```python
from build123d import *

# Parameters (mm, degrees)
BOSS_EXTRUDE1_DEPTH     = 25.4
CUT_EXTRUDE1_DEPTH      = 0.25399999999999945
CUT_EXTRUDE1_DEPTH_BACK = 3.8099999999999814
BOSS_EXTRUDE3_DEPTH     = 50.8
CUT_EXTRUDE3_DEPTH      = 38.1
SKETCH9_R               = 7.958201772862371
BOSS_EXTRUDE4_DEPTH     = 95.75799999999995
SKETCH11_W              = 88.91089611657237
SKETCH11_H              = 39.241441418777725
BOSS_EXTRUDE5_DEPTH     = 16.509999999999938
FILLET2_R               = 10
FILLET3_R               = 4.919999999999999


# Read off the part's stored shape, not the designer's step: Sweep1
with BuildPart() as part:
    # Sketch1 → Boss-Extrude1 (new body)
    with BuildSketch(Plane.XY):
        with BuildLine():
            Line((63.5, 77.01063829787236), (-63.5, 77.01063829787236))
            ThreePointArc((-63.5, 77.01063829787236), (-73.05346395858422, 73.05346395858422), (-77.01063829787236, 63.5))
            Line((-77.01063829787236, 63.5), (-77.01063829787236, -63.5))
            ThreePointArc((-77.01063829787236, -63.5), (-73.05346395858422, -73.05346395858422), (-63.5, -77.01063829787236))
            Line((-63.5, -77.01063829787236), (63.5, -77.01063829787236))
            ThreePointArc((63.5, -77.01063829787236), (73.05346395858422, -73.05346395858423), (77.01063829787236, -63.500000000000014))
            Line((77.01063829787236, -63.500000000000014), (77.01063829787236, 63.500000000000014))
            ThreePointArc((77.01063829787236, 63.500000000000014), (73.05346395858422, 73.05346395858423), (63.5, 77.01063829787236))
        make_face()
    extrude(amount=BOSS_EXTRUDE1_DEPTH)

    # Sketch3 → Cut-Extrude1 (cut, two sides: drawn at the far end of the back side and taken through both)
    with BuildSketch(Plane.XY.offset(25.4).offset(-CUT_EXTRUDE1_DEPTH_BACK)):
        with BuildLine():
            Line((-64.31063829787236, -55.89490495185724), (-64.31063829787236, 55.89490495185724))
            ThreePointArc((-64.31063829787236, 55.89490495185724), (-61.826342998624284, 61.86512188051967), (-55.84013695793273, 64.31063829787234))
            Line((-55.84013695793273, 64.31063829787234), (55.84013695793273, 64.31063829787234))
            ThreePointArc((55.84013695793273, 64.31063829787234), (61.826342998624284, 61.86512188051967), (64.31063829787236, 55.89490495185724))
            Line((64.31063829787236, 55.89490495185724), (64.31063829787236, -55.89490495185724))
            ThreePointArc((64.31063829787236, -55.89490495185724), (61.826342998624284, -61.86512188051967), (55.84013695793273, -64.31063829787234))
            Line((55.84013695793273, -64.31063829787234), (-55.84013695793273, -64.31063829787234))
            ThreePointArc((-55.84013695793273, -64.31063829787234), (-61.826342998624284, -61.86512188051967), (-64.31063829787236, -55.89490495185724))
        make_face()
    extrude(amount=CUT_EXTRUDE1_DEPTH + CUT_EXTRUDE1_DEPTH_BACK, mode=Mode.SUBTRACT)

    # Sketch7 → Boss-Extrude3 (add)
    with BuildSketch(Plane(origin=(0, 0, 0), x_dir=(-1, 0, 0), z_dir=(0, 0, -1))):
        with BuildLine():
            Line((-25.971736510678774, -77.01063829787236), (25.971736510678774, -77.0106382978723))
            Line((25.971736510678774, -77.0106382978723), (25.971736510678774, -33.11396405111534))
            ThreePointArc((25.971736510678774, -33.11396405111534), (-4.77e-15, -7.142227540436579), (-25.971736510678774, -33.11396405111537))
            Line((-25.971736510678774, -33.11396405111537), (-25.971736510678774, -77.01063829787236))
        make_face()
    extrude(amount=BOSS_EXTRUDE3_DEPTH)

    # Sketch8 → Cut-Extrude3 (cut)
    with BuildSketch(Plane(origin=(0, 0, -50.8), x_dir=(-1, 0, 0), z_dir=(0, 0, -1))):
        with BuildLine():
            Line((-10.388694604271498, -77.01063829787235), (-10.388694604271498, -31.815377225581233))
            ThreePointArc((-10.388694604271498, -31.815377225581233), (6.4e-16, -21.426682621309737), (10.388694604271498, -31.815377225581233))
            Line((10.388694604271498, -31.815377225581233), (10.388694604271498, -77.01063829787235))
            Line((10.388694604271498, -77.01063829787235), (-10.388694604271498, -77.01063829787235))
        make_face()
    extrude(amount=-CUT_EXTRUDE3_DEPTH, mode=Mode.SUBTRACT)

    # Sketch9 → Boss-Extrude4 (add)
    with BuildSketch(Plane(origin=(0, -19.311882184983943, -23.015004973711303), x_dir=(1, 0, 0), z_dir=(0, -0.6427876096865301, -0.7660444431189859))):
        with Locations(Location((0, 16.20859028637191, 0), (0, 0, 358.83868965))):
            Circle(SKETCH9_R)
    extrude(amount=BOSS_EXTRUDE4_DEPTH)



with BuildPart() as body_2:
    # Sketch11 → Boss-Extrude5 (new body)
    with BuildSketch(Plane(origin=(0, -80.86393811334668, -96.36988875789913), x_dir=(-1, 0, 0), z_dir=(0, -0.64278760968653, -0.766044443118986))):
        with Locations((0, -16.2085902863719)):
            Rectangle(SKETCH11_W, SKETCH11_H)
    extrude(amount=BOSS_EXTRUDE5_DEPTH)


with BuildPart() as part_1:
    add(part.part)

    add(body_2.part)  # Sweep1 merges body 2
    # Sweep1 outline → Sweep1 (revolve)
    with BuildSketch(Plane(origin=(0, -12.41650052, 10.418681007), x_dir=(1, 0, 0), z_dir=(0, -0.766044443118986, 0.64278760968653))):
        with BuildLine():
            ThreePointArc((14.308201773, -125.801955257), (12.448329834, -121.311827197), (7.958201773, -119.451955257))
            Line((7.958201773, -119.451955257), (7.958201773, -125.801955257))
            Line((7.958201773, -125.801955257), (14.308201773, -125.801955257))
        make_face()
    revolve(axis=Axis((0, -12.41650052, 10.418681007), (0, 0.64278760968653, 0.766044443118986)))

    # Fillet2
    # the kernel refuses this fillet: 10 mm, written as the material it takes off along each edge
    with BuildSketch(Plane(origin=(-55.894727894264214, 55.894904951857264, 25.4), x_dir=(-1, -2.53e-15, 0), z_dir=(2.53e-15, -1, 0))) as fillet2_piece_1:
        with BuildLine():
            CenterArc((16.269820257941824, 10), FILLET2_R, 218.24314589443497, 51.756854105565026)
            Line((8.415910403608144, 3.809999999999981), (8.258832206521468, 3.6861999999999817))
            ThreePointArc((8.258832206521468, 3.6861999999999817), (8.215910403608142, 1.9049999999999905), (8.215910403608142, 0))
            Line((8.215910403608142, 0), (8.415910403608144, -0.1999999999999993))
            Line((8.415910403608144, -0.1999999999999993), (16.269820257941824, -0.1999999999999993))
            Line((16.269820257941824, -0.1999999999999993), (16.269820257941824, 0))
        make_face()
    revolve(axis=Axis((-55.894727894264214, 55.894904951857264, 25.4), (0, 0, -1)), revolution_arc=90.37165939708579, mode=Mode.SUBTRACT)
    with BuildSketch(Plane(origin=(55.894727894264214, 55.894904951857264, 25.4), x_dir=(-0.00648663468518885, 0.9999789615639225, 0), z_dir=(-0.9999789615639225, -0.00648663468518885, 0))) as fillet2_piece_2:
        with BuildLine():
            CenterArc((16.269820257941824, 10), FILLET2_R, 218.24314589443495, 51.756854105565026)
            Line((8.415910403608141, 3.809999999999981), (8.258832206521465, 3.6861999999999817))
            ThreePointArc((8.258832206521465, 3.6861999999999817), (8.215910403608135, 1.9049999999999905), (8.215910403608135, 0))
            Line((8.215910403608135, 0), (8.415910403608141, -0.1999999999999993))
            Line((8.415910403608141, -0.1999999999999993), (16.269820257941824, -0.1999999999999993))
            Line((16.269820257941824, -0.1999999999999993), (16.269820257941824, 0))
        make_face()
    revolve(axis=Axis((55.894727894264214, 55.894904951857264, 25.4), (0, 0, -1)), revolution_arc=90.37165939708579, mode=Mode.SUBTRACT)
    with BuildSketch(Plane(origin=(64.31063829787236, -55.894904951857235, 25.4), x_dir=(1, 0, 0), z_dir=(0, 1, 0)), Plane(origin=(-64.31063829787236, 55.894904951857235, 25.4), x_dir=(-1, 0, 0), z_dir=(0, -1, 0))) as fillet2_piece_3:
        with BuildLine():
            CenterArc((7.853909854333679, 10), FILLET2_R, 218.24314589443497, 51.756854105565026)
            Line((0, 3.809999999999981), (-0.15707819708667614, 3.6861999999999817))
            ThreePointArc((-0.15707819708667614, 3.6861999999999817), (-0.20000000000000284, 1.9049999999999905), (-0.20000000000000284, 0))
            Line((-0.20000000000000284, 0), (0, -0.1999999999999993))
            Line((0, -0.1999999999999993), (7.853909854333679, -0.1999999999999993))
            Line((7.853909854333679, -0.1999999999999993), (7.853909854333679, 0))
        make_face()
    extrude(amount=111.78980990371448, mode=Mode.SUBTRACT)
    with BuildSketch(Plane(origin=(55.894727894264214, -55.894904951857264, 25.4), x_dir=(1, 2.53e-15, 0), z_dir=(-2.53e-15, 1, 0))) as fillet2_piece_4:
        with BuildLine():
            CenterArc((16.269820257941824, 10), FILLET2_R, 218.24314589443497, 51.756854105565026)
            Line((8.415910403608144, 3.809999999999981), (8.258832206521468, 3.6861999999999817))
            ThreePointArc((8.258832206521468, 3.6861999999999817), (8.215910403608142, 1.9049999999999905), (8.215910403608142, 0))
            Line((8.215910403608142, 0), (8.415910403608144, -0.1999999999999993))
            Line((8.415910403608144, -0.1999999999999993), (16.269820257941824, -0.1999999999999993))
            Line((16.269820257941824, -0.1999999999999993), (16.269820257941824, 0))
        make_face()
    revolve(axis=Axis((55.894727894264214, -55.894904951857264, 25.4), (0, 0, -1)), revolution_arc=90.37165939708579, mode=Mode.SUBTRACT)
    with BuildSketch(Plane(origin=(-55.840136957932735, -64.31063829787234, 25.4), x_dir=(0, -1, 0), z_dir=(1, 0, 0)), Plane(origin=(55.840136957932735, 64.31063829787234, 25.4), x_dir=(0, 1, 0), z_dir=(-1, 0, 0))) as fillet2_piece_5:
        with BuildLine():
            CenterArc((7.853909854333679, 10), FILLET2_R, 218.24314589443497, 51.756854105565026)
            Line((0, 3.809999999999981), (-0.15707819708667614, 3.6861999999999817))
            ThreePointArc((-0.15707819708667614, 3.6861999999999817), (-0.20000000000000284, 1.9049999999999905), (-0.20000000000000284, 0))
            Line((-0.20000000000000284, 0), (0, -0.1999999999999993))
            Line((0, -0.1999999999999993), (7.853909854333679, -0.1999999999999993))
            Line((7.853909854333679, -0.1999999999999993), (7.853909854333679, 0))
        make_face()
    extrude(amount=111.68027391586546, mode=Mode.SUBTRACT)
    with BuildSketch(Plane(origin=(-55.894727894264214, -55.894904951857264, 25.4), x_dir=(0.00648663468518885, -0.9999789615639225, 0), z_dir=(0.9999789615639225, 0.00648663468518885, 0))) as fillet2_piece_6:
        with BuildLine():
            CenterArc((16.269820257941824, 10), FILLET2_R, 218.24314589443495, 51.756854105565026)
            Line((8.415910403608141, 3.809999999999981), (8.258832206521465, 3.6861999999999817))
            ThreePointArc((8.258832206521465, 3.6861999999999817), (8.215910403608135, 1.9049999999999905), (8.215910403608135, 0))
            Line((8.215910403608135, 0), (8.415910403608141, -0.1999999999999993))
            Line((8.415910403608141, -0.1999999999999993), (16.269820257941824, -0.1999999999999993))
            Line((16.269820257941824, -0.1999999999999993), (16.269820257941824, 0))
        make_face()
    revolve(axis=Axis((-55.894727894264214, -55.894904951857264, 25.4), (0, 0, -1)), revolution_arc=90.37165939708579, mode=Mode.SUBTRACT)

    # Fillet3
    fillet3_edges = [part_1.edges().sort_by_distance(p)[0] for p in [
        (-44.45544805828619, -93.28043863301424, -85.95120775133383),
        (0, -78.2500945635973, -98.5631639164489),
        (44.45544805828619, -93.28043863301424, -85.95120775133383),
        (0, -108.3107827024312, -73.33925158621877),
    ]]
    fillet(fillet3_edges, radius=FILLET3_R)


solid = part_1.part
```
Part model, mm, in its own coordinate system. A direction names the side the tool comes from. Round coordinates to 2 decimals unless told otherwise and drop trailing zeros. Order: outer loops, then holes, each group sorted by start corner. A loop starts at its lowest first (then second) coordinate and runs counter-clockwise, first axis right, second up. Notation, with made-up numbers: M 15,37.5 L 30,37.5 A26 ccw 30,60.5 Z; hole C 66,31 d3. An arc over 180 degrees is marked long. Answer in a Markdown table with one row per item. Add a question column.
Q1. Mould opens along Z. For faces 1 (the face through (-0.17, -29.4, -14.55)), 2 (the face through (-73.158, -72.948, 12.522)), 3 (the face through (12, -42, -50.8)), 4 (the face through (3.53, -54.6, -50.95)) say: +Z half, -Z half, draft (parallel to the pull), parting line (faces both ways), or undercut.
Q2. Wall check: L1, parallel to Z at x = 52, y = 34.5; L2, parallel to Y at x = -7, z = 2; L3, parallel to Z at x = -16, y = -66. Give the ranges that are in metal, low to high. Write a range as from..to.
Q3. Pin check, flat tips, straight feed: pin 1 (4 mm diameter, centred on x = -38.5, y = -12, fed in from -Z); pin 2 (13 mm diameter, centred on y = -63, z = -17.5, fed in from -X); pin 3 (10 mm diameter, centred on x = -2.5, z = -35, fed in from +Y). Stop position of each tip, or through.
Q4. Cut at D-D on x = 0. Give the cut face in (y, z).
Q5. Cut at A-A on x = -36.5. Give the cut face in (y, z).
Q6. Cut at C-C on z = 8. Give the cut face in (x, y), and give its area (3 significant figures).
Q7. Cut at B-B on y = 13.5. Give the cut face in (x, z), and give its area (3 significant figures).
Q8. 3-axis set-ups, long thin cutter, end or side, ignore diameter. For faces 5 (the face through (-67.74, 0.78, 24.37)), 6 (the face through (-1, 1, 0)), 7 (the face through (-10.389, -54, -32)), 8 (the face through (-25.972, -55, -25)): which of +Z, -Z, +X, -X, +Y, -Y reach the whole face in a straight line?
Established:
| question | item | result |
|---|---|---|
| 1 | face 1 | undercut |
| 1 | face 2 | draft |
| 1 | face 3 | -Z half |
| 1 | face 4 | undercut |
| 2 | L1 | z = 0..21.59 |
| 2 | L2 | y = -77.01..77.01 |
| 2 | L3 | z = -50.8..23.27 |
| 3 | pin 1 | stops at z = 0 |
| 3 | pin 2 | stops at x = -25.97 |
| 3 | pin 3 | stops at y = -7.14 |
| 4 | outline | M -118.92,-85.99 L -88.86,-111.21 L -81.41,-102.33 A4.92 ccw -82.02,-95.4 L -82.32,-95.15 A6.35 ccw -83.1,-86.2 L -25.63,-17.71 L -31.6,-12.7 L -21.43,-12.7 L -21.43,-50.8 L -7.14,-50.8 L -7.14,0 L 77.01,0 L 77.01,25.4 L 72.16,25.4 A10 ccw 64.31,21.59 L -64.31,21.59 A10 ccw -72.16,25.4 L -77.01,25.4 L -77.01,-12.7 L -42.2,-12.7 L -95.3,-75.97 A6.35 ccw -104.24,-76.75 L -104.54,-76.5 A4.92 ccw -111.47,-77.11 Z |
| 5 | outline | M -118.92,-85.99 L -88.86,-111.21 L -81.41,-102.33 A4.92 ccw -82.02,-95.4 L -104.54,-76.5 A4.92 ccw -111.47,-77.11 Z; M -77.01,0 L 77.01,0 L 77.01,25.4 L 72.16,25.4 A10 ccw 64.31,21.59 L -64.31,21.59 A10 ccw -72.16,25.4 L -77.01,25.4 Z |
| 6 | outline | M -77.01,-63.5 A13.51 ccw -63.5,-77.01 L 63.5,-77.01 A13.51 ccw 77.01,-63.5 L 77.01,63.5 A13.51 ccw 63.5,77.01 L -63.5,77.01 A13.51 ccw -77.01,63.5 Z |
| 6 | area | 23,600 mm2 |
| 7 | outline | M -77.01,0 L 77.01,0 L 77.01,25.4 L 72.16,25.4 A10 ccw 64.31,21.59 L -64.31,21.59 A10 ccw -72.16,25.4 L -77.01,25.4 Z |
| 7 | area | 3,400 mm2 |
| 8 | face 5 | +Z |
| 8 | face 6 | -Z, +Y |
| 8 | face 7 | -Z, -Y |
| 8 | face 8 | -Z, -X, +Y, -Y |
